```python
from build123d import *

# Parameters (mm, degrees)
SKETCH1_W           = 90
SKETCH1_H           = 87
SKETCH1_W_2         = 12
SKETCH1_H_2         = 3
BOSS_EXTRUDE1_DEPTH = 3
SKETCH3_R           = 3
BOSS_EXTRUDE2_DEPTH = 3


with BuildPart() as part:
    # Sketch1 → Boss-Extrude1 (new body)
    with BuildSketch(Plane(origin=(0, 0, 0), x_dir=(1, 0, 0), z_dir=(0, 1, 0))):
        Rectangle(SKETCH1_W, SKETCH1_H)
        with Locations((30, 39)):
            Rectangle(SKETCH1_W_2, SKETCH1_H_2, mode=Mode.SUBTRACT)
    extrude(amount=BOSS_EXTRUDE1_DEPTH)

    # Sketch3 → Boss-Extrude2 (add)
    with BuildSketch(Plane.XY.offset(40.5)):
        with BuildLine():
            Line((24, 3), (24, 10))
            ThreePointArc((24, 10), (30, 16), (36, 10))
            Line((36, 10), (36, 3))
            Line((36, 3), (24, 3))
        make_face()
        with Locations((30, 10)):
            Circle(SKETCH3_R, mode=Mode.SUBTRACT)
    extrude(amount=-BOSS_EXTRUDE2_DEPTH)


solid = part.part
```
The listing builds one solid part. Answer for the finished solid, in the listing's coordinates (mm). A direction names the side the tool comes from. Give positions to 0.01 mm unless a question says otherwise; leave off trailing zeros. Loops run counter-clockwise (first coordinate to the right, second up) from the corner with the lowest first, then second, coordinate; pieces in that order, holes last. Notation, with made-up numbers: M -34.5,-38.75 L 15.5,-38.75 A19 ccw 15.5,-19.75 Z; hole C -29,-30.75 d5. An arc over 180 degrees is marked long. One line per item, written item: value.
1. For a pull along Z with two mould halves and no side action, classify faces 1 (the face through (30, 16, 39)), 2 (the face through (30, 1, -40.5)), 3 (the face through (-1, 1, -43.5)) as pulls with the +Z half, pulls with the -Z half, needs draft (parallel to the pull), parting line crosses it, or undercut.
Found:
face 1: needs draft
face 2: undercut
face 3: pulls with the -Z half
2. Section B-B on y = 8.25 is taken. Determine the outline of the cut face in (x, z).
Found:
outline: M 24,37.5 L 27.56,37.5 L 27.56,40.5 L 24,40.5 Z; M 32.44,37.5 L 36,37.5 L 36,40.5 L 32.44,40.5 Z
3. Section C-C on x = -24.5 is taken. Determine the outline of the cut face in (y, z).
Found:
outline: M 0,-43.5 L 3,-43.5 L 3,43.5 L 0,43.5 Z
4. For faces 4 (the face through (30.1, 6.7, 37.5)), 5 (the face through (30.1, 6.7, 40.5)), 6 (the face through (36, 7, 39)), 7 (the face through (30, 1, -37.5)), 8 (the face through (24, 6, 39)), determine the directions among +Z, -Z, +X, -X, +Y, -Y from which every point of the face is accessible in a straight line to the end or side of a thin tool.
Found:
face 4: -Z, +X, -X, +Y
face 5: +Z, +X, -X, +Y
face 6: +Z, -Z, +X, +Y
face 7: +Y, -Y
face 8: +Z, -Z, -X, +Y
5. Find the intervals of material crossed by probe 1 along Y at (x, z) = (30, 38.4); probe 2 along Y at (x, z) = (-18.5, 15); probe 3 along Z at (x, y) = (32.5, 5.75), in increasing order.
Found:
probe 1: 0 to 7, 13 to 16
probe 2: 0 to 3
probe 3: 37.5 to 40.5
6. Section D-D on z = -26.5 is taken. Determine the outline of the cut face in (x, y), plus the area to 3 significant figures.
Found:
outline: M -45,0 L 45,0 L 45,3 L -45,3 Z
area: 270 mm^2
7. Section A-A on x = 30 is taken. Determine the outline of the cut face in (y, z), plus the area to 3 significant figures.
Found:
outline: M 0,-43.5 L 3,-43.5 L 3,-40.5 L 0,-40.5 Z; M 0,-37.5 L 3,-37.5 L 3,37.5 L 7,37.5 L 7,40.5 L 3,40.5 L 3,43.5 L 0,43.5 Z; M 13,37.5 L 16,37.5 L 16,40.5 L 13,40.5 Z
area: 273 mm^2
8. Each of these flat-tipped pins is pushed along its axis until it touches: P1, Ø1, axis at x = 3, z = 23, coming from the +Y side; P2, Ø4, axis at y = 3.5, z = -11.5, coming from the -X side; P3, Ø2.5, axis at y = 7, z = 39.5, coming from the +X side; P4, Ø2.5, axis at y = 6, z = 38.5, coming from the -X side. Where does it stop, or does it pass through?
Found:
P1: y = 3
P2: x = -45
P3: x = 36
P4: x = 24
